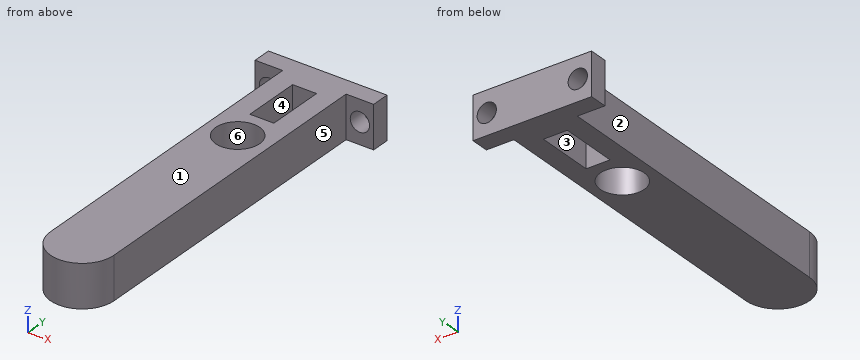
```python
from build123d import *

# Parameters (mm, degrees)
ESTRUSIONE_ESTRUSIONE3_DEPTH = 15.5
SCHIZZO6_R                   = 8
TAGLIO_ESTRUSIONE1_DEPTH     = 15.5
SCHIZZO7_W                   = 8.7
SCHIZZO7_H                   = 21.146442976
TAGLIO_ESTRUSIONE2_DEPTH     = 15.5
SCHIZZO14_R                  = 3.5
TAGLIO_ESTRUSIONE3_DEPTH     = 6.6
SCHIZZO15_R                  = 3.5
TAGLIO_ESTRUSIONE4_DEPTH     = 6.6


with BuildPart() as part:
    # Schizzo3 → Estrusione-Estrusione3 (new body)
    with BuildSketch(Plane.XY):
        with BuildLine():
            Line((-62.60213075, -3.859058403), (-62.60213075, 111.140941597))
            Line((-62.60213075, 111.140941597), (-72.60213075, 111.140941597))
            Line((-72.60213075, 111.140941597), (-72.60213075, 117.740941597))
            Line((-72.60213075, 117.740941597), (-29.60213075, 117.740941597))
            Line((-29.60213075, 117.740941597), (-29.60213075, 111.140941597))
            Line((-29.60213075, 111.140941597), (-39.60213075, 111.140941597))
            Line((-39.60213075, 111.140941597), (-39.60213075, -3.859058403))
            ThreePointArc((-39.60213075, -3.859058403), (-51.10213075, -15.359058403), (-62.60213075, -3.859058403))
        make_face()
    extrude(amount=ESTRUSIONE_ESTRUSIONE3_DEPTH)

    # Schizzo6 → Taglio-Estrusione1 (cut)
    with BuildSketch(Plane.XY):
        with Locations((-51.10213075, 73.140941597)):
            Circle(SCHIZZO6_R)
    extrude(amount=TAGLIO_ESTRUSIONE1_DEPTH, mode=Mode.SUBTRACT)

    # Schizzo7 → Taglio-Estrusione2 (cut)
    with BuildSketch(Plane.XY):
        with Locations((-51.10213075, 95.714163085)):
            Rectangle(SCHIZZO7_W, SCHIZZO7_H)
    extrude(amount=TAGLIO_ESTRUSIONE2_DEPTH, mode=Mode.SUBTRACT)

    # Schizzo14 → Taglio-Estrusione3 (cut)
    with BuildSketch(Plane(origin=(0, 111.140941597, 0), x_dir=(-1, 0, 0), z_dir=(0, -1, 0))):
        with Locations(Location((34.60213075, -7.75, 0), (0, 0, 90))):
            Circle(SCHIZZO14_R)
    extrude(amount=-TAGLIO_ESTRUSIONE3_DEPTH, mode=Mode.SUBTRACT)

    # Schizzo15 → Taglio-Estrusione4 (cut)
    with BuildSketch(Plane(origin=(0, 111.140941597, 0), x_dir=(-1, 0, 0), z_dir=(0, -1, 0))):
        with Locations(Location((67.60213075, -7.75, 0), (0, 0, 90))):
            Circle(SCHIZZO15_R)
    extrude(amount=-TAGLIO_ESTRUSIONE4_DEPTH, mode=Mode.SUBTRACT)


solid = part.part
```
Geometry: final body of the model. Coordinates: model frame, mm. Face numbers are marked on the shaded views. A direction names the side the tool comes from. Round coordinates to 2 decimals unless told otherwise and drop trailing zeros. Write each loop counter-clockwise with the first axis right and the second up, starting at its lowest first coordinate (ties: lowest second). Pieces come first, ordered by that corner, then holes.
Item 1: Pin query (flat end, axial travel): P1, Ø4.5, axis at x = -52, z = 10.5, coming from the -Y side; P2, Ø8, axis at y = 76, z = 13.5, coming from the +X side; P3, Ø8, axis at y = 89, z = 4.5, coming from the -X side; P4, Ø4, axis at x = -47.5, z = 3.5, coming from the -Y side. Return the tip coordinate at first contact, or that it passes through.
Item 2: Section query B-B (x = -51). Return loops of the section in (y, z), plus the area to 3 significant figures.
Item 3: Material intervals for L1, parallel to X at y = 93.5, z = 7; L2, parallel to Y at x = -54, z = 6.25; L3, parallel to X at y = 31, z = 6.5, sorted ascending.
Item 4: Section query A-A (z = 7.75). Return loops of the section in (x, y).
Item 5: Set-up query: the marked faces 5 and 6. Return all of +Z, -Z, +X, -X, +Y, -Y with unobstructed straight access to the full face (end or side cutting, diameter ignored); none if empty.
Item 6: Section query C-C (z = 1.5). Return loops of the section in (x, y), plus the area to 3 significant figures.
Item 7: Mould query, pull axis X, two halves, no side actions, for the marked faces 1, 2, 3 and 4. Classes: +X half, -X half, draft (parallel to the pull), parting line (faces both ways), or undercut.
Item 8: Section query D-D (y = 42.5). Return loops of the section in (x, z), plus the area to 4 significant figures.
Completed:
1. P1: stops at y = -15.36
1. P2: stops at x = -39.6
1. P3: stops at x = -62.6
1. P4: stops at y = -15.25
2. outline: (-15.36, 0) - (65.14, 0) - (65.14, 15.5) - (-15.36, 15.5) - close; (81.14, 0) - (85.14, 0) - (85.14, 15.5) - (81.14, 15.5) - close; (106.29, 0) - (117.74, 0) - (117.74, 15.5) - (106.29, 15.5) - close
2. area: 1,490 mm2
3. L1: x = -62.6 to -55.45, -46.75 to -39.6
3. L2: y = -14.99 to 65.68, 80.6 to 85.14, 106.29 to 117.74
3. L3: x = -62.6 to -39.6
4. outline: (-72.6, 111.14) - (-71.1, 111.14) - (-71.1, 117.74) - (-72.6, 117.74) - close; (-64.1, 111.14) - (-62.6, 111.14) - (-62.6, -3.86) arc R11.5 ccw to (-39.6, -3.86) - (-39.6, 111.14) - (-38.1, 111.14) - (-38.1, 117.74) - (-64.1, 117.74) - close; (-31.1, 111.14) - (-29.6, 111.14) - (-29.6, 117.74) - (-31.1, 117.74) - close; hole circle Ø16 at (-51.1, 73.14); hole (-55.45, 85.14) - (-46.75, 85.14) - (-46.75, 106.29) - (-55.45, 106.29) - close
5. face 5: +Z, -Z, +X, -Y
5. face 6: +Z, -Z
6. outline: (-72.6, 111.14) - (-62.6, 111.14) - (-62.6, -3.86) arc R11.5 ccw to (-39.6, -3.86) - (-39.6, 111.14) - (-29.6, 111.14) - (-29.6, 117.74) - (-72.6, 117.74) - close; hole circle Ø16 at (-51.1, 73.14); hole (-55.45, 85.14) - (-46.75, 85.14) - (-46.75, 106.29) - (-55.45, 106.29) - close
6. area: 2,750 mm2
7. face 1: draft
7. face 2: -X half
7. face 3: undercut
7. face 4: undercut
8. outline: (-62.6, 0) - (-39.6, 0) - (-39.6, 15.5) - (-62.6, 15.5) - close
8. area: 356.5 mm2
